Input: part model. Units: mm. Frame: model coordinates. Give positions to 0.01 mm unless a question says otherwise; leave off trailing zeros. Loops run counter-clockwise (first coordinate to the right, second up) from the corner with the lowest first, then second, coordinate; pieces in that order, holes last. Notation, with made-up numbers: M 58.5,-8.75 L 83.5,-8.75 A26 ccw 83.5,6.25 Z; hole C 67,-28 d10. An arc over 180 degrees is marked long. Use CSV: the item, a comma, the result in double quotes. Start each with the question number.
Q1. Pull-direction query (Z, two-part tool) for faces 1 (the flat face through (0, 1, -30)), 2 (the cylindrical face through (0.1, 1.5, -13.1)), 3 (the cylindrical face through (0.28, 1.462, 30.195)), 4 (the flat face through (-20, 2, 0)); classes: released by +Z, released by -Z, zero draft, split by the parting line, or undercut.
Q2. Section A-A, the plane z = -10. Output: boundary loops of the cut face in (x, y), plus the area to 3 significant figures.
Q3. Section C-C, the plane y = 2.05. Output: boundary loops of the cut face in (x, z).
Q4. Section B-B, the plane x = 0. Output: boundary loops of the cut face in (y, z) (3 decimals).
Q5. Material intervals for line 1 along X through (y, z) = (1.5, -10); line 2 along Z through (x, y) = (-1.5, 0.55); line 3 along Z through (x, y) = (-14.5, 2.3), sorted ascending.
from build123d import *

# Parameters (mm, degrees)
SKETCH1_W           = 40
SKETCH1_H           = 60
SKETCH1_R           = 3.1
BOSS_EXTRUDE1_DEPTH = 3
BOSS_EXTRUDE2_DEPTH = 40


with BuildPart() as part:
    # Sketch1 → Boss-Extrude1 (new body)
    with BuildSketch(Plane(origin=(0, 0, 0), x_dir=(1, 0, 0), z_dir=(0, 1, 0))):
        Rectangle(SKETCH1_W, SKETCH1_H)
        with Locations(Location((0, 10, 0), (0, 0, 270))):
            Circle(SKETCH1_R, mode=Mode.SUBTRACT)
    extrude(amount=BOSS_EXTRUDE1_DEPTH)

    # Sketch3 → Boss-Extrude2 (add)
    with BuildSketch(Plane(origin=(20, 0, 0), x_dir=(0, 0, -1), z_dir=(1, 0, 0))):
        with BuildLine():
            Line((-30, 0), (-30.562875043, 0))
            ThreePointArc((-30.562875043, 0), (-30.190981376, 1.483028164), (-30, 3))
            Line((-30, 3), (-30, 0))
        make_face()
    extrude(amount=-BOSS_EXTRUDE2_DEPTH)


solid = part.part
A:
1,face 1,"released by -Z"
1,face 2,"undercut"
1,face 3,"released by +Z"
1,face 4,"zero draft"
2,outline,"M -20,0 L -3.1,0 L -3.1,3 L -20,3 Z; M 3.1,0 L 20,0 L 20,3 L 3.1,3 Z"
2,area,"101 mm^2"
3,outline,"M -20,-30 L 20,-30 L 20,30.1 L -20,30.1 Z; hole C 0,-10 d6.2"
4,outline,"M 0,-30 L 3,-30 L 3,-13.1 L 0,-13.1 Z; M 0,-6.9 L 3,-6.9 L 3,30 A12.7 cw 0,30.563 Z"
5,line 1,"-20 to -3.1, 3.1 to 20"
5,line 2,"-30 to -12.71, -7.29 to 30.4"
5,line 3,"-30 to 30.07"
